Source: CAD feature listing. Evaluate the final solid. Frame: model axes, mm. A direction names the side the tool comes from. Give positions to 0.01 mm unless a question says otherwise; leave off trailing zeros. Write each loop counter-clockwise with the first axis right and the second up, starting at its lowest first coordinate (ties: lowest second). Pieces come first, ordered by that corner, then holes.
```python
from build123d import *

# Parameters (mm, degrees)
SKETCH1_W           = 50
SKETCH1_H           = 36
SKETCH1_R           = 4
BOSS_EXTRUDE1_DEPTH = 12
CUT_EXTRUDE1_REACH  = 47.442
SKETCH2_R           = 3


with BuildPart() as part:
    # Sketch1 → Boss-Extrude1 (new body)
    with BuildSketch(Plane.XY):
        Rectangle(SKETCH1_W, SKETCH1_H)
        with Locations((-15, 8)):
            Circle(SKETCH1_R, mode=Mode.SUBTRACT)
        with Locations((-15, -8)):
            Circle(SKETCH1_R, mode=Mode.SUBTRACT)
        with Locations((15, -8)):
            Circle(SKETCH1_R, mode=Mode.SUBTRACT)
        with Locations((15, 8)):
            Circle(SKETCH1_R, mode=Mode.SUBTRACT)
    extrude(amount=BOSS_EXTRUDE1_DEPTH)

    # Sketch2 → Cut-Extrude1 (cut, up to next)
    with BuildSketch(Plane(origin=(0, 18, 0), x_dir=(1, 0, 0), z_dir=(0, 1, 0)), mode=Mode.PRIVATE) as cut_extrude1_sk1:
        with Locations(Location((-15, -6, 0), (0, 0, 270))):
            Circle(SKETCH2_R)
    cut_extrude1_tool1 = extrude(cut_extrude1_sk1.sketch, amount=-CUT_EXTRUDE1_REACH, mode=Mode.PRIVATE) & part.part
    # Sketch2 → Cut-Extrude1 (cut, up to next)
    with BuildSketch(Plane(origin=(0, 18, 0), x_dir=(1, 0, 0), z_dir=(0, 1, 0)), mode=Mode.PRIVATE) as cut_extrude1_sk2:
        with Locations(Location((15, -6, 0), (0, 0, 270))):
            Circle(SKETCH2_R)
    cut_extrude1_tool2 = extrude(cut_extrude1_sk2.sketch, amount=-CUT_EXTRUDE1_REACH, mode=Mode.PRIVATE) & part.part
    cut_extrude1_1 = cut_extrude1_tool1.solids().sort_by_distance((-15, 18, 6))[0]
    add(cut_extrude1_1, mode=Mode.SUBTRACT)
    cut_extrude1_2 = cut_extrude1_tool2.solids().sort_by_distance((15, 18, 6))[0]
    add(cut_extrude1_2, mode=Mode.SUBTRACT)
    cut_extrude1 = cut_extrude1_1 + cut_extrude1_2  # Cut-Extrude1 as one shape, for the pattern or mirror that repeats it

    # Mirror1: Cut-Extrude1 across plane
    add(cut_extrude1.mirror(Plane.ZX), mode=Mode.SUBTRACT)


solid = part.part
```
1. Mould query, pull axis X, two halves, no side actions, for faces 1 (the flat face through (-25, 0, 6)), 2 (the flat face through (0, -18, 6)), 3 (the cylindrical face through (13.85, -14.37, 8.77)), 4 (the cylindrical face through (-16.15, 14.37, 8.77)). Classes: +X half, -X half, draft (parallel to the pull), parting line (faces both ways), or undercut.
2. Cut plane D-D, the plane y = 5. Return the cut outline in (x, z), then the cut area to 3 significant figures.
3. Cut plane A-A, the plane z = 1. Return the cut outline in (x, y), then the cut area to 3 significant figures.
4. Access query for faces 5 (the cylindrical face through (13.85, 14.37, 8.77)), 6 (the cylindrical face through (-16.15, -14.37, 8.77)), 7 (the flat face through (0, 18, 6)). Directions: +Z, -Z, +X, -X, +Y, -Y. A direction counts if a zero-diameter tool reaches every point of the face in a straight line with its end or side. Return the directions, or none.
5. Contact query for flat-ended pins moving along their axis: P1, Ø3.5, axis at x = -15, z = 6, coming from the +Y side; P2, Ø3.5, axis at x = 15, z = 6, coming from the -Y side. Output: stop coordinate, or through.
6. Line query: L1, parallel to X at y = 15.5, z = 6; L2, parallel to Z at x = -15, y = -14; L3, parallel to X at y = 7, z = 3.5. Output: solid intervals per line, ascending.
7. Cut plane B-B, the plane x = 15. Return the cut outline in (y, z).
8. Cut plane C-C, the plane y = 15. Return the cut outline in (x, z).
Response values:
1. face 1: -X half
1. face 2: draft
1. face 3: undercut
1. face 4: undercut
2. outline: (-25, 0) - (-17.65, 0) - (-17.65, 12) - (-25, 12) - close; (-12.35, 0) - (12.35, 0) - (12.35, 12) - (-12.35, 12) - close; (17.65, 0) - (25, 0) - (25, 12) - (17.65, 12) - close
2. area: 473 mm2
3. outline: (-25, -18) - (25, -18) - (25, 18) - (-25, 18) - close; hole circle Ø8 at (-15, -8); hole circle Ø8 at (-15, 8); hole circle Ø8 at (15, -8); hole circle Ø8 at (15, 8)
3. area: 1,600 mm2
4. face 5: +Y
4. face 6: -Y
4. face 7: +Z, -Z, +X, -X, +Y
5. P1: stops at y = 4.4
5. P2: stops at y = -4.4
6. L1: x = -25 to -18, -12 to 12, 18 to 25
6. L2: z = 0 to 3, 9 to 12
6. L3: x = -25 to -18.87, -11.13 to 11.13, 18.87 to 25
7. outline: (-18, 0) - (-12, 0) - (-12, 3) - (-18, 3) - close; (-18, 9) - (-12, 9) - (-12, 12) - (-18, 12) - close; (-4, 0) - (4, 0) - (4, 12) - (-4, 12) - close; (12, 0) - (18, 0) - (18, 3) - (12, 3) - close; (12, 9) - (18, 9) - (18, 12) - (12, 12) - close
8. outline: (-25, 0) - (25, 0) - (25, 12) - (-25, 12) - close; hole circle Ø6 at (-15, 6); hole circle Ø6 at (15, 6)
